CAD build for the part. Positions are in the model's coordinates, mm. Face numbers are marked on the shaded views. A direction names the side the tool comes from. Give positions to 0.01 mm unless a question says otherwise; leave off trailing zeros. Loops run counter-clockwise (first coordinate to the right, second up) from the corner with the lowest first, then second, coordinate; pieces in that order, holes last. Notation, with made-up numbers: M 33.25,-28.5 L 59.25,-28.5 A8 cw 59.25,-18.5 Z; hole C 68,84.25 d10. An arc over 180 degrees is marked long. Answer as CSV lines item,"result".
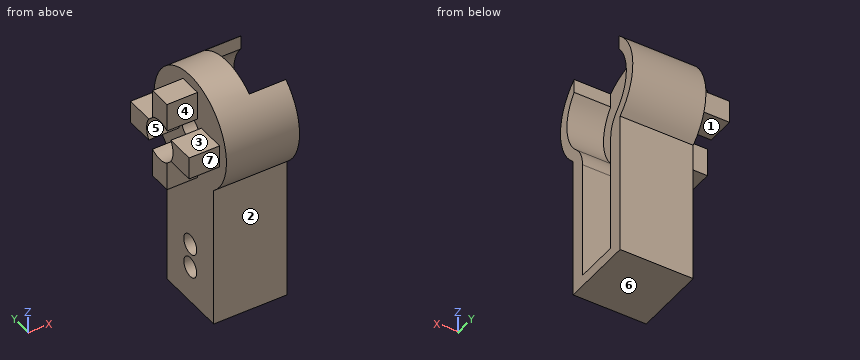
from build123d import *

# Parameters (mm, degrees)
BOSS_EXTRUDE1_DEPTH = 12
SKETCH2_R           = 7.6
SKETCH2_W           = 22
SKETCH2_H           = 7.2
SKETCH2_W_2         = 6.090233647
SKETCH2_H_2         = 11.5
CUT_EXTRUDE1_DEPTH  = 6
FILLET1_R           = 5
SKETCH3_R           = 2.25
SKETCH3_R_2         = 1.65
CUT_EXTRUDE2_DEPTH  = 6
BOSS_EXTRUDE2_DEPTH = 5
SKETCH6_R           = 3.375
CUT_EXTRUDE3_DEPTH  = 5


with BuildPart() as part:
    # Sketch1 → Boss-Extrude1 (new body)
    with BuildSketch(Plane(origin=(0, 0, 0), x_dir=(0, 0, -1), z_dir=(1, 0, 0))):
        with BuildLine():
            Line((30.54006392, 6), (7.04006392, 6))
            ThreePointArc((7.04006392, 6), (8.679950785, 3.197022735), (9.25, 0))
            ThreePointArc((9.25, 0), (8.679950785, -3.197022735), (7.04006392, -6))
            Line((7.04006392, -6), (30.54006392, -6))
            Line((30.54006392, -6), (30.54006392, 6))
        make_face()
        with BuildLine():
            ThreePointArc((9.25, 0), (8.679950785, 3.197022735), (7.04006392, 6))
            Line((7.04006392, 6), (7.04006392, -6))
            ThreePointArc((7.04006392, -6), (8.679950785, -3.197022735), (9.25, 0))
        make_face()
        with BuildLine():
            Line((7.04006392, -6), (7.04006392, 6))
            ThreePointArc((7.04006392, 6), (-9.25, 0), (7.04006392, -6))
        make_face()
    extrude(amount=BOSS_EXTRUDE1_DEPTH)

    # Sketch2 → Cut-Extrude1 (cut)
    with BuildSketch(Plane(origin=(12, 0, 0), x_dir=(0, 0, -1), z_dir=(1, 0, 0))):
        Circle(SKETCH2_R)
        with Locations((17.693280212, 0)):
            Rectangle(SKETCH2_W, SKETCH2_H)
        with Locations((-8.014774759, 0)):
            Rectangle(SKETCH2_W_2, SKETCH2_H_2)
    extrude(amount=-CUT_EXTRUDE1_DEPTH, mode=Mode.SUBTRACT)

    # Fillet1
    fillet1_edges = [part.edges().sort_by_distance(p)[0] for p in [
        (9, 3.6, -6.693280212),
        (9, -3.6, -6.693280212),
    ]]
    fillet(fillet1_edges, radius=FILLET1_R)

    # Sketch3 → Cut-Extrude2 (cut)
    with BuildSketch(Plane(origin=(6, 0, 0), x_dir=(0, 0, -1), z_dir=(1, 0, 0))):
        Circle(SKETCH3_R)
        with Locations((20.5, 0)):
            Circle(SKETCH3_R_2)
        with Locations((24.5, 0)):
            Circle(SKETCH3_R_2)
    extrude(amount=-CUT_EXTRUDE2_DEPTH, mode=Mode.SUBTRACT)

    # Sketch5 → Boss-Extrude2 (add)
    with BuildSketch(Plane.ZY):
        with BuildLine():
            Line((-1.85, 1.85), (-7.5, 1.85))
            Line((-7.5, 1.85), (-7.5, -1.85))
            Line((-7.5, -1.85), (-1.85, -1.85))
            Line((-1.85, -1.85), (-1.85, -1.280624847))
            ThreePointArc((-1.85, -1.280624847), (-2.25, 0), (-1.85, 1.280624847))
            Line((-1.85, 1.280624847), (-1.85, 1.85))
        make_face()
        with BuildLine():
            Line((-1.85, 7.5), (-1.85, 1.85))
            Line((-1.85, 1.85), (-1.280624847, 1.85))
            ThreePointArc((-1.280624847, 1.85), (0, 2.25), (1.280624847, 1.85))
            Line((1.280624847, 1.85), (1.85, 1.85))
            Line((1.85, 1.85), (1.85, 7.5))
            Line((1.85, 7.5), (-1.85, 7.5))
        make_face()
        with BuildLine():
            Line((7.5, 1.85), (1.85, 1.85))
            Line((1.85, 1.85), (1.85, 1.280624847))
            ThreePointArc((1.85, 1.280624847), (2.147673159, 0.670820393), (2.25, 0))
            ThreePointArc((2.25, 0), (2.147673159, -0.670820393), (1.85, -1.280624847))
            Line((1.85, -1.280624847), (1.85, -1.85))
            Line((1.85, -1.85), (7.5, -1.85))
            Line((7.5, -1.85), (7.5, 1.85))
        make_face()
        with BuildLine():
            Line((-1.280624847, -1.85), (-1.85, -1.85))
            Line((-1.85, -1.85), (-1.85, -7.5))
            Line((-1.85, -7.5), (1.85, -7.5))
            Line((1.85, -7.5), (1.85, -1.85))
            Line((1.85, -1.85), (1.280624847, -1.85))
            ThreePointArc((1.280624847, -1.85), (0, -2.25), (-1.280624847, -1.85))
        make_face()
        with BuildLine():
            Line((-1.280624847, 1.85), (-1.85, 1.85))
            Line((-1.85, 1.85), (-1.85, 1.280624847))
            ThreePointArc((-1.85, 1.280624847), (-1.590990258, 1.590990258), (-1.280624847, 1.85))
        make_face()
        with BuildLine():
            Line((1.85, 1.85), (1.280624847, 1.85))
            ThreePointArc((1.280624847, 1.85), (1.590990258, 1.590990258), (1.85, 1.280624847))
            Line((1.85, 1.280624847), (1.85, 1.85))
        make_face()
        with BuildLine():
            ThreePointArc((1.85, -1.280624847), (1.590990258, -1.590990258), (1.280624847, -1.85))
            Line((1.280624847, -1.85), (1.85, -1.85))
            Line((1.85, -1.85), (1.85, -1.280624847))
        make_face()
        with BuildLine():
            Line((-1.85, -1.280624847), (-1.85, -1.85))
            Line((-1.85, -1.85), (-1.280624847, -1.85))
            ThreePointArc((-1.280624847, -1.85), (-1.590990258, -1.590990258), (-1.85, -1.280624847))
        make_face()
    extrude(amount=BOSS_EXTRUDE2_DEPTH)

    # Sketch6 → Cut-Extrude3 (cut)
    with BuildSketch(Plane.ZY.offset(5)):
        Circle(SKETCH6_R)
    extrude(amount=-CUT_EXTRUDE3_DEPTH, mode=Mode.SUBTRACT)


solid = part.part
1) Drill centre lines: line 1 (Y direction, x = 3.95, z = -20.5); line 2 (Y direction, x = 6.5, z = -14.5); line 3 (Y direction, x = -1.5, z = 6.5). Where is each one in solid material? Low to high. Write a range as from..to.
Answer below:
line 1,"y = -6..-1.65, 1.65..6"
line 2,"y = -6..-3.6, 3.6..6"
line 3,"y = -1.85..1.85"
2) Mould opens along Z. For the marked faces 5, 6 and 7 say: +Z half, -Z half, draft (parallel to the pull), parting line (faces both ways), or undercut.
Answer below:
face 5,"undercut"
face 6,"-Z half"
face 7,"draft"
3) Flat gauge pins, fed straight in: pin 1 (1 mm diameter, centred on x = 9.5, z = -26.5, fed in from -Y); pin 2 (1.4 mm diameter, centred on x = -3.5, z = 6, fed in from -Y); pin 3 (5.5 mm diameter, centred on y = 0, z = -20.5, fed in from -X); pin 4 (2 mm diameter, centred on y = 0, z = -24.5, fed in from -X). Where does each tip first touch, or does it go through?
Answer below:
pin 1,"stops at y = -6"
pin 2,"stops at y = -1.85"
pin 3,"stops at x = 0"
pin 4,"passes through"
4) Band-saw the part on B-B on x = -3. Give the cut face in (y, z) (3 decimals), and give its area (3 significant figures).
Answer below:
outline,"M -7.5,-1.85 L -2.823,-1.85 A3.375 cw -2.823,1.85 L -7.5,1.85 Z; M -1.85,-7.5 L 1.85,-7.5 L 1.85,-2.823 A3.375 cw -1.85,-2.823 Z; M -1.85,2.823 A3.375 cw 1.85,2.823 L 1.85,7.5 L -1.85,7.5 Z; M 2.823,-1.85 L 7.5,-1.85 L 7.5,1.85 L 2.823,1.85 A3.375 cw Z"
area,"63.7 mm^2"
5) Which spindle directions (+Z, -Z, +X, -X, +Y, -Y) get a long thin tool onto all of the face, cutting with end or side? Do the marked faces 1, 2, 3 and 4. Say none if no direction does.
Answer below:
face 1,"-Z, -X, +Y, -Y"
face 2,"-Z, +X, -X, -Y"
face 3,"+Z, -X, +Y, -Y"
face 4,"+Z, -Z, -X, -Y"
6) Band-saw the part on C-C on y = 0. Give the cut face in (x, z) (3 decimals).
Answer below:
outline,"M -5,-7.5 L 0,-7.5 L 0,-18.85 L 6,-18.85 L 6,-2.25 L 0,-2.25 L 0,-3.375 L -5,-3.375 Z; M -5,3.375 L 0,3.375 L 0,2.25 L 6,2.25 L 6,9.25 L 0,9.25 L 0,7.5 L -5,7.5 Z; M 0,-30.54 L 12,-30.54 L 12,-28.693 L 6,-28.693 L 6,-26.15 L 0,-26.15 Z; M 0,-22.85 L 6,-22.85 L 6,-22.15 L 0,-22.15 Z"
7) Band-saw the part on A-A on z = 0. Give the cut face in (x, y) (3 decimals).
Answer below:
outline,"M -5,-7.5 L 0,-7.5 L 0,-9.25 L 12,-9.25 L 12,-7.6 L 6,-7.6 L 6,-2.25 L 0,-2.25 L 0,-3.375 L -5,-3.375 Z; M -5,3.375 L 0,3.375 L 0,2.25 L 6,2.25 L 6,7.6 L 12,7.6 L 12,9.25 L 0,9.25 L 0,7.5 L -5,7.5 Z"
8) Band-saw the part on D-D on z = -10. Give the cut face in (x, y), and give its area (3 significant figures).
Answer below:
outline,"M 0,-6 L 12,-6 L 12,-3.6 L 6,-3.6 L 6,3.6 L 12,3.6 L 12,6 L 0,6 Z"
area,"101 mm^2"
